Geometry check sheet. Reference: the model listing, model coordinates, mm. Face numbers are marked on the shaded views. A direction names the side the tool comes from. Coordinates: 2 decimals unless noted, no trailing zeros. Write each loop counter-clockwise with the first axis right and the second up, starting at its lowest first coordinate (ties: lowest second). Pieces come first, ordered by that corner, then holes. Notation, with made-up numbers: M 60.25,85 L 98.25,85 A28 cw 98.25,116 Z; hole C 25.25,-40 d3. An arc over 180 degrees is marked long. Put each result on its own line as item: value. Start each with the question number.
1) Mould release check, pull along X, two halves, no side actions. Record for the marked faces 3, 4 and 5: released by +X, released by -X, zero draft, split by the parting line, or undercut.
2) Scan lines: line 1 along X through (y, z) = (0.7, 0) (3 decimals); line 2 along X through (y, z) = (-0.6, 0); line 3 along Z through (x, y) = (0.25, 0.85). Record each from-to range of solid material in increasing order.
3) Set-up check for the marked faces 1 and 2: record each of +Z, -Z, +X, -X, +Y, -Y from which the full face is reachable in a straight line by a thin tool's end or side.
4) Cross-section at D-D on y = -0.4. Record the cut outline in (x, z).
5) Cross-section at B-B on y = 1. Record the cut outline in (x, z) (3 decimals).
6) Cross-section at A-A on x = 0. Record the cut outline in (y, z) (3 decimals), plus the area to 3 significant figures.
7) Gauge pin test, flat end, axial feed: pin 1 (4 mm diameter, centred on x = -7.25, z = 0, fed in from -Y). Record the tip position at first contact, or that the pin passes through.
8) Cross-section at C-C on z = 0.75. Count the separate pieces of the cut face and the enclosed holes in it, plus the area to 3 significant figures.
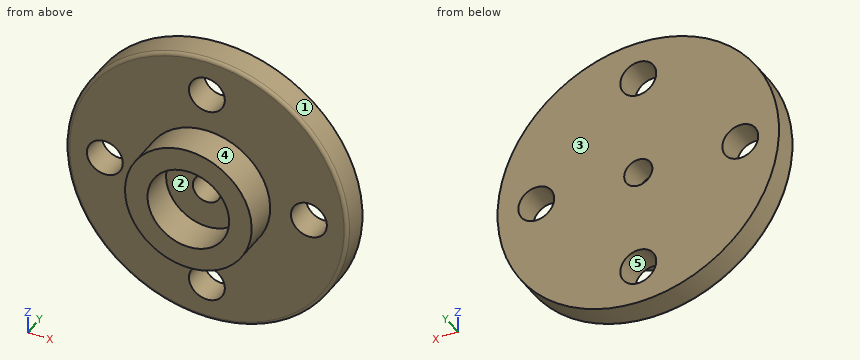
from build123d import *

# Parameters (mm, degrees)
SKETCH1_R           = 10
BOSS_EXTRUDE1_DEPTH = 2
SKETCH2_R           = 4.5
BOSS_EXTRUDE2_DEPTH = 2.5
SKETCH3_R           = 1.275
CUT_EXTRUDE1_DEPTH  = 15.361406616
FILLET1_R           = 0.25
SKETCH6_R           = 1
CUT_EXTRUDE2_DEPTH  = 15.840822214
SKETCH7_R           = 2.9
CUT_EXTRUDE3_DEPTH  = 2.5


with BuildPart() as part:
    # Sketch1 → Boss-Extrude1 (new body)
    with BuildSketch(Plane(origin=(0, 0, 0), x_dir=(1, 0, 0), z_dir=(0, 1, 0))):
        with Locations(Location((0, 0, 0), (0, 0, 270))):
            Circle(SKETCH1_R)
    extrude(amount=BOSS_EXTRUDE1_DEPTH)

    # Sketch2 → Boss-Extrude2 (add)
    with BuildSketch(Plane(origin=(0, 0, 0), x_dir=(1, 0, 0), z_dir=(0, 1, 0))):
        with Locations(Location((0, 0, 0), (0, 0, 270))):
            Circle(SKETCH2_R)
    extrude(amount=-BOSS_EXTRUDE2_DEPTH)

    # Sketch3 → Cut-Extrude1 (cut, through all)
    with BuildSketch(Plane(origin=(0, 0, 0), x_dir=(1, 0, 0), z_dir=(0, 1, 0))):
        with Locations(Location((0, 7.25, 0), (0, 0, 270))):
            Circle(SKETCH3_R)
        with Locations(Location((-7.25, 0, 0), (0, 0, 270))):
            Circle(SKETCH3_R)
        with Locations(Location((0, -7.25, 0), (0, 0, 90))):
            Circle(SKETCH3_R)
        with Locations(Location((7.25, 0, 0), (0, 0, 90))):
            Circle(SKETCH3_R)
    extrude(amount=CUT_EXTRUDE1_DEPTH, mode=Mode.SUBTRACT)

    # Fillet1
    fillet1_edges = [part.edges().sort_by_distance(p)[0] for p in [
        (0, 0, -10),
    ]]
    fillet(fillet1_edges, radius=FILLET1_R)

    # Sketch6 → Cut-Extrude2 (cut, through all)
    with BuildSketch(Plane(origin=(0, 2, 0), x_dir=(1, 0, 0), z_dir=(0, 1, 0))):
        with Locations(Location((0, 0, 0), (0, 0, 270))):
            Circle(SKETCH6_R)
    extrude(amount=-CUT_EXTRUDE2_DEPTH, mode=Mode.SUBTRACT)

    # Sketch7 → Cut-Extrude3 (cut)
    with BuildSketch(Plane.XZ.offset(2.5)):
        with Locations(Location((0, 0, 0), (0, 0, 270))):
            Circle(SKETCH7_R)
    extrude(amount=-CUT_EXTRUDE3_DEPTH, mode=Mode.SUBTRACT)


solid = part.part
Answer key:
1. face 3: zero draft
1. face 4: split by the parting line
1. face 5: undercut
2. line 1: x = -10 to -8.525, -5.975 to -1, 1 to 5.975, 8.525 to 10
2. line 2: x = -4.5 to -2.9, 2.9 to 4.5
2. line 3: z = -10 to -8.5, -6 to -0.97, 0.97 to 6, 8.5 to 10
3. face 1: +Y, -Y
3. face 2: -Y
4. outline: C 0,0 d9; hole C 0,0 d5.8
5. outline: C 0,0 d20; hole C -7.25,0 d2.55; hole C 0,-7.25 d2.55; hole C 0,7.25 d2.55; hole C 0,0 d2; hole C 7.25,0 d2.55
6. outline: M -2.5,-4.5 L 0,-4.5 L 0,-5.975 L 2,-5.975 L 2,-1 L 0,-1 L 0,-2.9 L -2.5,-2.9 Z; M -2.5,2.9 L 0,2.9 L 0,1 L 2,1 L 2,5.975 L 0,5.975 L 0,4.5 L -2.5,4.5 Z; M 0,-9.75 A0.25 ccw 0.25,-10 L 2,-10 L 2,-8.525 L 0,-8.525 Z; M 0,8.525 L 2,8.525 L 2,10 L 0.25,10 A0.25 ccw 0,9.75 Z
6. area: 33.8 mm²
7. pin 1: stops at y = 0
8. separate pieces: 4
8. enclosed holes: 0
8. area: 37.1 mm²
